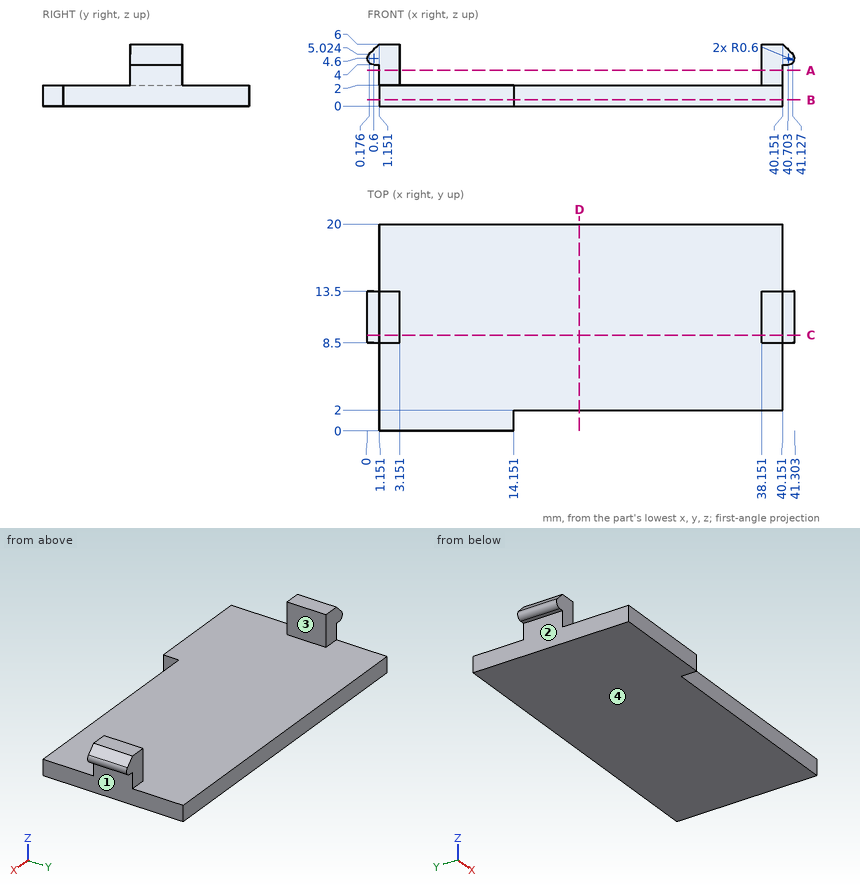
Can you work these out from the drawing? Everything is in mm from the part's minimum corner. A direction names the side the tool comes from. Coordinates: 2 decimals unless noted, no trailing zeros. Loops run counter-clockwise (first coordinate to the right, second up) from the corner with the lowest first, then second, coordinate; pieces in that order, holes last.
1) Imagine slicing it at A-A on z = 3.45. List the corners of the cut face in (x, y) for me, plus the area to 3 significant figures.
2) For pin 1 (0.9 mm diameter, centred on x = 2.5, z = 3.5, fed in from -Y); pin 2 (3 mm diameter, centred on x = 18, y = 6, fed in from +Z); pin 3 (2 mm diameter, centred on y = 9.5, z = 1.5, fed in from +X), each with a flat end and sliding along its axis, tell me the tip position at first contact or that it passes through.
3) Imagine slicing it at C-C on y = 9.25. List the corners of the cut face in (x, z) for me (1 decimal).
4) Imagine slicing it at B-B on z = 0.6. List the corners of the cut face in (x, y) for me.
5) I need wall thicknesses on probe 1 along Z at (x, y) = (8, 16.75); probe 2 along X at (y, z) = (9, 1.85); probe 3 along X at (y, z) = (10, 5.65). Which ranges of each line are inside material? Lowest first, please.
6) Which directions (+Z, -Z, +X, -X, +Y, -Y) give clear straight access to the entire face, cutting with the end or side of a thin tool? Please do the marked faces 1, 2, 3 and 4.
7) Imagine slicing it at D-D on x = 20.5. List the corners of the cut face in (y, z) for me.
Completed:
1. outline: (1.15, 8.5) - (3.15, 8.5) - (3.15, 13.5) - (1.15, 13.5) - close; (38.15, 8.5) - (40.15, 8.5) - (40.15, 13.5) - (38.15, 13.5) - close
1. area: 20.0 mm2
2. pin 1: stops at y = 8.5
2. pin 2: stops at z = 2
2. pin 3: stops at x = 40.15
3. outline: (0.2, 5) arc R0.6 ccw to (0.6, 4) - (1.2, 4) - (1.2, 0) - (40.2, 0) - (40.2, 4) - (40.7, 4) arc R0.6 ccw to (41.1, 5) - (40.2, 6) - (38.2, 6) - (38.2, 2) - (3.2, 2) - (3.2, 6) - (1.2, 6) - close
4. outline: (1.15, 0) - (14.15, 0) - (14.15, 2) - (40.15, 2) - (40.15, 20) - (1.15, 20) - close
5. probe 1: z = 0 to 2
5. probe 2: x = 1.15 to 40.15
5. probe 3: x = 0.8 to 3.15, 38.15 to 40.5
6. face 1: -Z, +X, +Y, -Y
6. face 2: -Z, -X, +Y, -Y
6. face 3: +Z, +Y, -Y
6. face 4: -Z, +X, -X, +Y, -Y
7. outline: (2, 0) - (20, 0) - (20, 2) - (2, 2) - close
